The drawing under review shows one solid part. Ordinate dimensions are in mm from its lowest x, y, z. A direction names the side the tool comes from. Round coordinates to 2 decimals unless told otherwise and drop trailing zeros. Order: outer loops, then holes, each group sorted by start corner. A loop starts at its lowest first (then second) coordinate and runs counter-clockwise, first axis right, second up. Notation, with made-up numbers: M -34,57.5 L -11,57.5 A21 cw -11,75.5 Z; hole C -30,37.5 d7. An arc over 180 degrees is marked long. Answer as a JSON object with one key per item and string values. Group by question number.
1) The part is to be moulded in two halves that separate along Y. For the marked faces 3, 4, 5 and 6, say which applies: +Y half, -Y half, draft (parallel to the pull), parting line (faces both ways), or undercut.
2) Insertion check: pin 1 Ø1 at (x, y) = (36.5, 71) entering from +Z; pin 2 Ø2 at (x, z) = (45.5, 18.5) entering from -Y; pin 3 Ø5 at (x, z) = (28, 3.5) entering from +Y. Each pin has a flat end and moves straight along its axis. Give the tip position at first contact, or say it passes through.
3) Consider section A-A, the plane z = 13. Write out the cut boundary in (x, y).
4) For the marked faces 1 and 2, list the 3-axis set-ups (+Z, -Z, +X, -X, +Y, -Y) from which the entire face can be reached by the end or side of a thin tool; tool diameter is ignored.
5) Consider section C-C, the plane z = 3.5. Write out the cut boundary in (x, y), then the cut area to 3 significant figures.
6) Consider section B-B, the plane x = 59.5. Count the separate pieces of the cut face and the enclosed holes in it.
7) To check wall thickness, follow line 1 (Y direction, x = 42, z = 19.25); line 2 (Z direction, x = 43, y = 79.5); line 3 (X direction, y = 58, z = 19.5) (1 decimal). State the ranges of each line that lie inside material, in increasing order.
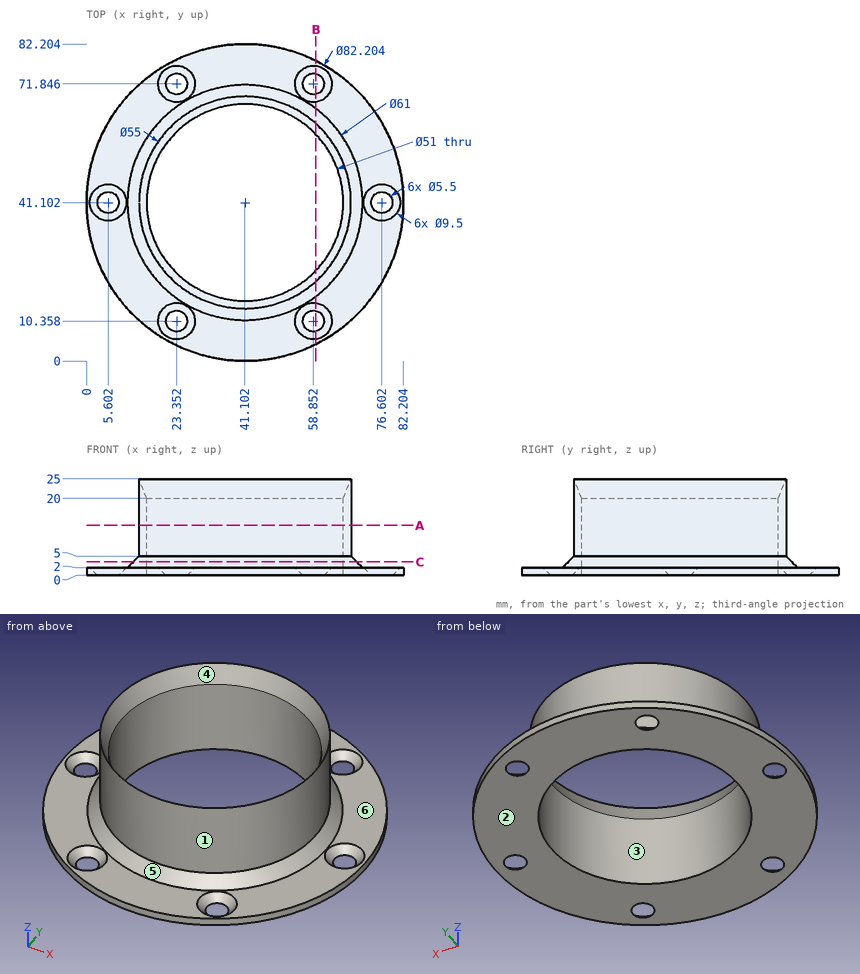
Results list:
{
 "1": {"face 3": "undercut", "face 4": "undercut", "face 5": "parting line", "face 6": "draft"},
 "2": {"pin 1": "z = 2.75", "pin 2": "y = 13.81", "pin 3": "y = 80.68"},
 "3": {"outline": "C 41.1,41.1 d55; hole C 41.1,41.1 d51"},
 "4": {"face 1": "+Z", "face 2": "-Z, +X, -X, +Y, -Y"},
 "5": {"outline": "C 41.1,41.1 d58; hole C 41.1,41.1 d51", "area": "599 mm^2"},
 "6": {"separate pieces": "4", "enclosed holes": "0"},
 "7": {"line 1": "13.62 to 15.62, 66.59 to 68.59", "line 2": "0 to 2", "line 3": "19.4 to 22, 60.2 to 62.8"}
}
